from build123d import *

# Parameters (mm, degrees)
SKETCH033_R        = 1.2
SKETCH033_R_2      = 1.764044
PAD020_DEPTH       = 3
PAD029_DEPTH       = 10.8
SKETCH046_R        = 1.7
POCKET003022_DEPTH = 20


with BuildPart() as part:
    # Sketch033 → Pad020 (new body)
    with BuildSketch(Plane.XY):
        with BuildLine():
            Line((35.5, 0), (35.5, 6.415183))
            ThreePointArc((35.988725, 49.947313), (33.757449, 28.203554), (35.5, 6.415183))
            ThreePointArc((35.988725, 49.947313), (36.349691, 66.784913), (32.171358, 83.099833))
            ThreePointArc((32.171358, 83.099833), (31.269586, 84.821896), (29.723476, 86.000133))
            Line((12.328447, 86.000133), (29.723476, 86.000133))
            ThreePointArc((0, 81.7771), (6.566085, 82.715448), (12.328447, 86.000133))
            Line((0, 81.7771), (0, 9.7771))
            ThreePointArc((9.7771, 0), (6.913454, 6.913454), (0, 9.7771))
            Line((35.5, 0), (9.7771, 0))
        make_face()
        with Locations((2.350144, 20.802189)):
            Circle(SKETCH033_R, mode=Mode.SUBTRACT)
        with Locations((21.7765, 43.6923)):
            Circle(SKETCH033_R, mode=Mode.SUBTRACT)
        with Locations((11.788759, 55.9729)):
            Circle(SKETCH033_R_2, mode=Mode.SUBTRACT)
        with Locations((31.788759, 55.9729)):
            Circle(SKETCH033_R_2, mode=Mode.SUBTRACT)
        with Locations((21.493771, 30)):
            Circle(SKETCH033_R_2, mode=Mode.SUBTRACT)
        Polygon((27.914344, 27.302489), (4.407844, 27.302489), (4.407844, 14.365089), (27.914344, 14.365089), (27.914344, 18.365089), (30.714344, 18.365089), (30.714344, 23.302489), (27.914344, 23.302489), align=None, mode=Mode.SUBTRACT)
        with BuildLine():
            Line((15.2762, 68.75), (15.2762, 45.75))
            Line((15.2762, 45.75), (28.2136, 45.75))
            Line((28.2136, 45.75), (28.2136, 68.75))
            Line((24.2136, 68.75), (28.2136, 68.75))
            ThreePointArc((24.2136, 68.75), (21.7449, 71.728653), (19.2762, 68.75))
            Line((15.2762, 68.75), (19.2762, 68.75))
        make_face(mode=Mode.SUBTRACT)
    extrude(amount=PAD020_DEPTH)

    # Sketch045 → Pad029 (new body)
    with BuildSketch(Plane.XY.offset(3)):
        with BuildLine():
            Line((16.768312, 79.999998), (16.768312, 86))
            Line((16.768312, 86), (26.122612, 86))
            Line((26.122612, 79.999999), (26.122612, 86))
            ThreePointArc((16.768312, 79.999998), (21.445462, 75.32285), (26.122612, 79.999999))
        make_face()
    extrude(amount=PAD029_DEPTH)

    # Sketch046 → Pocket003022 (cut)
    with BuildSketch(Plane.XY.offset(13.8)):
        with Locations((21.445462, 80)):
            Circle(SKETCH046_R)
    extrude(amount=-POCKET003022_DEPTH, mode=Mode.SUBTRACT)


solid = part.part
The listing builds one solid part. Answer for the finished solid, in the listing's coordinates (mm). A direction names the side the tool comes from. Coordinates: 2 decimals unless noted, no trailing zeros. Order: outer loops, then holes, each group sorted by start corner. A loop starts at its lowest first (then second) coordinate and runs counter-clockwise, first axis right, second up. Notation, with made-up numbers: (-4.75, 45.25) -> (41.25, 45.25) arc R21 ccw to (41.25, 83.25) -> close; hole circle Ø5 at (0.25, 17). An arc over 180 degrees is marked (long way). Answer in a Markdown table with one row per item. Add a question column.
Item 1: Which of the six approach directions +Z, -Z, +X, -X, +Y, -Y give full straight-line access (tool end or side, diameter ignored) to faces 1 (the face through (0, 46, 1)), 2 (the face through (29, 18.365, 1))?
Item 2: Find the intervals of material crossed by L1, parallel to Y at x = 22.5, z = 1; L2, parallel to X at y = 80, z = 5.5; L3, parallel to Z at x = 32.5, y = 24, in increasing order. Write a range as from..to.
Item 3: Determine the mould class of faces 3 (the face through (21.807, 71.728, 1.479)), 4 (the face through (6.989, 6.837, 1.479)), 5 (the face through (33.76, 28.51, 1.48)) for opening direction X: +X half, -X half, draft (parallel to the pull), parting line (faces both ways), or undercut.
Item 4: Find section B-B (y = 26). Write down the section's boundary in (x, z), then the cut area to 3 significant figures.
Item 5: Each of these flat-tipped pins is pushed along its axis until it touches: P1, Ø0.9, axis at y = 52, z = 2, coming from the +X side; P2, Ø2.5, axis at y = 23, z = 1.5, coming from the +X side; P3, Ø18.5, axis at x = 26.5, y = 34.5, coming from the +Z side. Where does it stop, or does it pass through?
Item 6: Find section C-C (z = 1.5). State how many separate pieces and enclosed holes the cut face has, then the cut area to 3 significant figures.
Item 7: Find section D-D (y = 12.5). Write down the section's boundary in (x, z), then the cut area to 3 significant figures.
Result set:
| question | item | result |
|---|---|---|
| 1 | face 1 | +Z, -Z, -X, +Y, -Y |
| 1 | face 2 | +Z, -Z |
| 2 | L1 | y = 0..14.37, 27.3..28.55, 31.45..42.73, 44.65..45.75, 71.61..78.67, 81.33..86 |
| 2 | L2 | x = 16.77..19.75, 23.15..26.12 |
| 2 | L3 | z = 0..3 |
| 3 | face 3 | undercut |
| 3 | face 4 | -X half |
| 3 | face 5 | +X half |
| 4 | outline | (0, 0) -> (4.41, 0) -> (4.41, 3) -> (0, 3) -> close; (27.91, 0) -> (33.75, 0) -> (33.75, 3) -> (27.91, 3) -> close |
| 4 | area | 30.7 mm² |
| 5 | P1 | stops at x = 36.33 |
| 5 | P2 | stops at x = 33.86 |
| 5 | P3 | stops at z = 3 |
| 6 | separate pieces | 1 |
| 6 | enclosed holes | 8 |
| 6 | area | 2,210 mm² |
| 7 | outline | (0, 0) -> (34.61, 0) -> (34.61, 3) -> (0, 3) -> close |
| 7 | area | 104 mm² |
